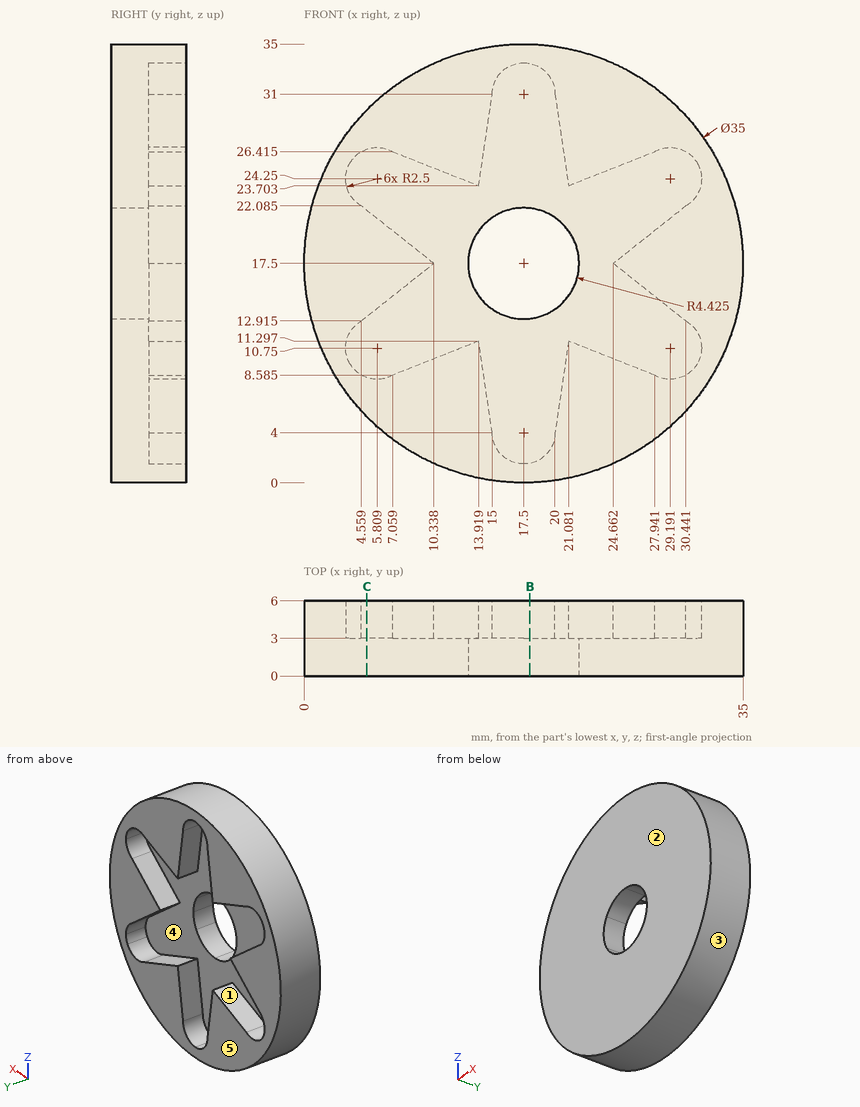
Design review of the part shown in the three views and the two pictorial views. Dimensions are in mm from the part's minimum x, y and z. A direction names the side the tool comes from. Give positions to 0.01 mm unless a question says otherwise; leave off trailing zeros. Write each loop counter-clockwise with the first axis right and the second up, starting at its lowest first coordinate (ties: lowest second). Pieces come first, ordered by that corner, then holes. Notation, with made-up numbers: (32.25, 48.25) -> (73.25, 48.25) arc R24 cw to (73.25, 73.25) -> close; hole circle Ø4 at (-32, -5). An arc over 180 degrees is marked (long way). Answer in a Markdown table with one row per item.
1) For L1, parallel to Z at x = 5, y = 5.7 (1 decimal); L2, parallel to Z at x = 10, y = 4.8; L3, parallel to Y at x = 23, z = 12.5, list the stretches that pass through material, from the lowest coordinate up. Write a range as [from, to].
Worked answers:
| item | result |
|---|---|
| L1 | [5.3, 8.4], [13.3, 21.7], [26.6, 29.7] |
| L2 | [1.69, 9.75], [17.23, 17.77], [25.25, 33.31] |
| L3 | [0, 3] |
2) Mouldability with a two-part tool opening along X and no side actions: class the marked faces 3, 4 and 5 as +X half, -X half, draft (parallel to the pull), parting line (faces both ways), or undercut.
Worked answers:
| item | result |
|---|---|
| face 3 | parting line |
| face 4 | undercut |
| face 5 | draft |
3) Clearance check with flat-ended pins moving along their axes: P1, Ø1, axis at y = 5, z = 22, coming from the -X side; P2, Ø1, axis at x = 19.5, z = 27.5, coming from the +Y side; P3, Ø1, axis at x = 11, z = 25.5, coming from the -Y side; P4, Ø3, axis at y = 0.5, z = 22, coming from the +X side. State where each tip first meets the part, or that it passes through.
Worked answers:
| item | result |
|---|---|
| P1 | x = 0.46 |
| P2 | y = 3 |
| P3 | y = 0 |
| P4 | x = 34.74 |
4) Tool access review of the marked faces 1 and 2: name each direction out of +Z, -Z, +X, -X, +Y, -Y from which nothing blocks a thin tool from reaching the whole face with its end or side.
Worked answers:
| item | result |
|---|---|
| face 1 | +Y |
| face 2 | +Z, -Z, +X, -X, -Y |
5) Add section C-C on x = 5. State the section outline as (y, z) points (1 decimal).
Worked answers:
| item | result |
|---|---|
| outline | (0, 5.3) -> (6, 5.3) -> (6, 8.4) -> (3, 8.4) -> (3, 13.3) -> (6, 13.3) -> (6, 21.7) -> (3, 21.7) -> (3, 26.6) -> (6, 26.6) -> (6, 29.7) -> (0, 29.7) -> close |
6) Add section B-B on x = 18. State the section outline as (y, z) points.
Worked answers:
| item | result |
|---|---|
| outline | (0, 0.01) -> (6, 0.01) -> (6, 1.55) -> (3, 1.55) -> (3, 13.1) -> (0, 13.1) -> close; (0, 21.9) -> (3, 21.9) -> (3, 33.45) -> (6, 33.45) -> (6, 34.99) -> (0, 34.99) -> close |
